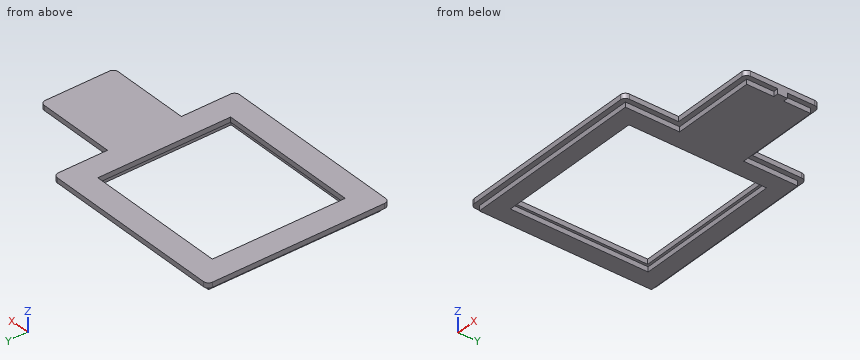
```python
from build123d import *

# Parameters (mm, degrees)
PAD_DEPTH            = 5
POCKET_DEPTH         = 4
SKETCH001_W          = 30
SKETCH001_H          = 28
PAD001_DEPTH         = 5
SKETCH003_W          = 29
SKETCH003_H          = 27
POCKET001_DEPTH      = 5
SKETCH004_W          = 2
SKETCH004_H          = 2
POCKET002_DEPTH      = 4
FILLET002_R          = 1
FILLET003_R          = 1
PAD002_DEPTH         = 2
SKETCH006_W          = 29
SKETCH006_H          = 27
POCKET003_DEPTH      = 0.001
POCKET003_DEPTH_BACK = -6.001
FILLET_R             = 1


with BuildPart() as body:
    # Sketch → Pad (new body)
    with BuildSketch(Plane.XY):
        Polygon((36.5, 7.5), (19.5, 7.5), (19.5, 18.5), (-19.5, 18.5), (-19.5, -18.5), (19.5, -18.5), (19.5, -7.5), (36.5, -7.5), align=None)
    extrude(amount=PAD_DEPTH)

    # Sketch002 → Pocket (cut)
    with BuildSketch(Plane.XY.offset(1)):
        Polygon((35.5, 6.5), (18.5, 6.5), (18.5, 17.5), (-18.5, 17.5), (-18.5, -17.5), (18.5, -17.5), (18.5, -6.5), (35.5, -6.5), align=None)
    extrude(amount=POCKET_DEPTH, mode=Mode.SUBTRACT)

    # Sketch001 → Pad001 (join)
    with BuildSketch(Plane.XY):
        Rectangle(SKETCH001_W, SKETCH001_H)
    extrude(amount=PAD001_DEPTH)

    # Sketch003 → Pocket001 (cut)
    with BuildSketch(Plane.XY):
        Rectangle(SKETCH003_W, SKETCH003_H)
    extrude(amount=POCKET001_DEPTH, mode=Mode.SUBTRACT)

    # Sketch004 → Pocket002 (cut)
    with BuildSketch(Plane.XY.offset(1)):
        with Locations((35.5, 0)):
            Rectangle(SKETCH004_W, SKETCH004_H)
    extrude(amount=POCKET002_DEPTH, mode=Mode.SUBTRACT)

    # Fillet002
    fillet002_edges = [body.edges().sort_by_distance(p)[0] for p in [
        (36.5, 7.5, 2.5),
        (19.5, 18.5, 2.5),
        (-19.5, 18.5, 2.5),
    ]]
    fillet(fillet002_edges, radius=FILLET002_R)

    # Fillet003
    fillet003_edges = [body.edges().sort_by_distance(p)[0] for p in [
        (36.5, -7.5, 2.5),
        (19.5, -18.5, 2.5),
        (-19.5, -18.5, 2.5),
    ]]
    fillet(fillet003_edges, radius=FILLET003_R)


with BuildPart() as cut:
    # Sketch005 → Pad002 (new body)
    with BuildSketch(Plane.XY.offset(4)):
        Polygon((36.5, 7.5), (19.5, 7.5), (19.5, 18.5), (-19.5, 18.5), (-19.5, -18.5), (19.5, -18.5), (19.5, -7.5), (36.5, -7.5), align=None)
    extrude(amount=PAD002_DEPTH)

    # Sketch006 → Pocket003 (cut, two sides)
    with BuildSketch(Plane.XY) as pocket003_sk:
        Rectangle(SKETCH006_W, SKETCH006_H)
    extrude(amount=-POCKET003_DEPTH, mode=Mode.SUBTRACT)
    extrude(pocket003_sk.sketch, amount=-POCKET003_DEPTH_BACK, mode=Mode.SUBTRACT)

    # Fillet
    fillet_edges = [cut.edges().sort_by_distance(p)[0] for p in [
        (36.5, -7.5, 5),
        (36.5, 7.5, 5),
        (19.5, 18.5, 5),
        (19.5, -18.5, 5),
        (-19.5, -18.5, 5),
        (-19.5, 18.5, 5),
    ]]
    fillet(fillet_edges, radius=FILLET_R)

    # Cut: cut Body
    add(body.part, mode=Mode.SUBTRACT)


solid = cut.part
```
For this review, take the finished solid that the model builds, in its own axes (mm). Give positions to 0.01 mm unless a question says otherwise; leave off trailing zeros. Write each loop counter-clockwise with the first axis right and the second up, starting at its lowest first coordinate (ties: lowest second). Pieces come first, ordered by that corner, then holes. Notation, with made-up numbers: M 75.5,36.25 L 95.5,36.25 A17 ccw 95.5,59.25 Z; hole C 42.5,75.25 d8. An arc over 180 degrees is marked long. One line per item, written item: value.
1) Take a section at D-D, the plane x = 27. Write out the cut boundary in (y, z).
Results are:
outline: M -7.5,5 L -6.5,5 L -6.5,4 L 6.5,4 L 6.5,5 L 7.5,5 L 7.5,6 L -7.5,6 Z
2) For P1, Ø0.8, axis at x = 2, z = 4.5, coming from the -Y side; P2, Ø0.8, axis at x = 36, z = 4.5, coming from the +Y side; P3, Ø0.5, axis at x = 25.5, z = 4.5, coming from the +Y side, all flat-tipped, find the tip position at first contact; note any pin that passes through.
Results are:
P1: stops at y = -17.5
P2: stops at y = 1
P3: stops at y = 6.5
3) Take a section at B-B, the plane x = -9.5. Write out the cut boundary in (y, z), then the cut area to 3 significant figures.
Results are:
outline: M -18.5,5 L -17.5,5 L -17.5,4 L -14,4 L -14,5 L -13.5,5 L -13.5,6 L -18.5,6 Z; M 13.5,5 L 14,5 L 14,4 L 17.5,4 L 17.5,5 L 18.5,5 L 18.5,6 L 13.5,6 Z
area: 17.0 mm²
4) Take a section at A-A, the plane z = 5.5. Write out the cut boundary in (x, y).
Results are:
outline: M -19.5,-17.5 A1 ccw -18.5,-18.5 L 18.5,-18.5 A1 ccw 19.5,-17.5 L 19.5,-7.5 L 35.5,-7.5 A1 ccw 36.5,-6.5 L 36.5,6.5 A1 ccw 35.5,7.5 L 19.5,7.5 L 19.5,17.5 A1 ccw 18.5,18.5 L -18.5,18.5 A1 ccw -19.5,17.5 Z; hole M -14.5,-13.5 L 14.5,-13.5 L 14.5,13.5 L -14.5,13.5 Z
5) Take a section at C-C, the plane y = -8.5. Write out the cut boundary in (x, z), then the cut area to 3 significant figures.
Results are:
outline: M -19.5,5 L -18.5,5 L -18.5,4 L -15,4 L -15,5 L -14.5,5 L -14.5,6 L -19.5,6 Z; M 14.5,5 L 15,5 L 15,4 L 18.5,4 L 18.5,5 L 19.5,5 L 19.5,6 L 14.5,6 Z
area: 17.0 mm²
6) For line 1 (Y direction, x = -12, z = 5.75); line 2 (X direction, y = -8, z = 5.1); line 3 (Y direction, x = 2, z = 4.25), list the stretches that pass through material, from the lowest coordinate up. Write a range as from..to.
Results are:
line 1: y = -18.5..-13.5, 13.5..18.5
line 2: x = -19.5..-14.5, 14.5..19.5
line 3: y = -17.5..-14, 14..17.5
